```python
from build123d import *

# Parameters (mm, degrees)
SKETCH1_R           = 1.5
BOSS_EXTRUDE1_DEPTH = 3
SKETCH4_W           = 27
SKETCH4_H           = 30
BOSS_EXTRUDE2_DEPTH = 2
SKETCH5_W           = 26
SKETCH5_H           = 30
BOSS_EXTRUDE3_DEPTH = 14
FILLET1_R           = 3


with BuildPart() as part:
    # Sketch1 → Boss-Extrude1 (new body)
    with BuildSketch(Plane.XY):
        Polygon((-14.5, 16), (14.5, 16), (22, 0), (14.5, -16), (-14.5, -16), (-22, 0), align=None)
        with Locations((-18, 0)):
            Circle(SKETCH1_R, mode=Mode.SUBTRACT)
        with Locations((18, 0)):
            Circle(SKETCH1_R, mode=Mode.SUBTRACT)
    extrude(amount=BOSS_EXTRUDE1_DEPTH)

    # Sketch4 → Boss-Extrude2 (add)
    with BuildSketch(Plane.XY.offset(3)):
        Rectangle(SKETCH4_W, SKETCH4_H)
    extrude(amount=BOSS_EXTRUDE2_DEPTH)

    # Sketch5 → Boss-Extrude3 (add)
    with BuildSketch(Plane(origin=(0, 0, 0), x_dir=(-1, 0, 0), z_dir=(0, 0, -1))):
        Rectangle(SKETCH5_W, SKETCH5_H)
    extrude(amount=BOSS_EXTRUDE3_DEPTH)

    # Fillet1
    fillet1_edges = [part.edges().sort_by_distance(p)[0] for p in [
        (-14.5, 16, 1.5),
        (14.5, 16, 1.5),
        (22, 0, 1.5),
        (14.5, -16, 1.5),
        (-14.5, -16, 1.5),
        (-22, 0, 1.5),
        (13.5, -15, 4),
        (13.5, 15, 4),
        (-13.5, 15, 4),
        (-13.5, -15, 4),
        (-13, -15, -7),
        (-13, 15, -7),
        (13, 15, -7),
        (13, -15, -7),
    ]]
    fillet(fillet1_edges, radius=FILLET1_R)


solid = part.part
```
The listing builds one solid part. Answer for the finished solid, in the listing's coordinates (mm). A direction names the side the tool comes from. Round coordinates to 2 decimals unless told otherwise and drop trailing zeros. Order: outer loops, then holes, each group sorted by start corner. A loop starts at its lowest first (then second) coordinate and runs counter-clockwise, first axis right, second up. Notation, with made-up numbers: (-9.75, 64.5) -> (23.25, 64.5) arc R14 ccw to (23.25, 82.5) -> close; hole circle Ø6 at (29.25, 65). An arc over 180 degrees is marked (long way). Answer as CSV lines item,"result". Start each with the question number.
(1) Flat-ended cylindrical pins translate along their axes: pin 1 Ø1 at (x, y) = (15, 5) entering from +Z; pin 2 Ø5 at (y, z) = (12.5, -4) entering from -X; pin 3 Ø11 at (x, z) = (-4, -6.5) entering from +Y. Find the tip coordinate at first contact, or state that the pin passes through.
(2) Find the intervals of material crossed by probe 1 along Z at (x, y) = (15, 2.5); probe 2 along X at (y, z) = (3, 4.25); probe 3 along X at (y, z) = (5, -1), in increasing order. Write a range as from..to.
(3) The part is cut by section C-C (y = -8). Determine the outline of the cut face in (x, z).
(4) The part is cut by section D-D (z = -3). Determine the outline of the cut face in (x, y), then the cut area to 3 significant figures.
(5) For a pull along X with two mould halves and no side action, classify faces 1 (the face through (0, -15, -7)), 2 (the face through (16.5, 0.07, 1.48)), 3 (the face through (12.1, 14.14, -7.1)) as +X half, -X half, draft (parallel to the pull), parting line (faces both ways), or undercut.
(6) The part is cut by section A-A (y = 0). Determine the outline of the cut face in (x, z), then the cut area to 3 significant figures.
(7) The part is cut by section B-B (x = 18). Determine the outline of the cut face in (y, z), then the cut area to 3 significant figures.
(8) A tool of negligible diameter and unlimited length cuts with its end or side. For faces 4 (the face through (0, -15, 4)), 5 (the face through (-13, 0, -7)), 6 (the face through (-13.5, 0, 4)), from which of +Z, -Z, +X, -X, +Y, -Y can it reach the whole face along a straight path? Write none if from no direction.
Evaluation:
1,pin 1,"z = 3"
1,pin 2,"x = -13"
1,pin 3,"y = 15"
2,probe 1,"0..3"
2,probe 2,"-13.5..13.5"
2,probe 3,"-13..13"
3,outline,"(-18.25, 0) -> (-13, 0) -> (-13, -14) -> (13, -14) -> (13, 0) -> (18.25, 0) -> (18.25, 3) -> (13.5, 3) -> (13.5, 5) -> (-13.5, 5) -> (-13.5, 3) -> (-18.25, 3) -> close"
4,outline,"(-13, -12) arc R3 ccw to (-10, -15) -> (10, -15) arc R3 ccw to (13, -12) -> (13, 12) arc R3 ccw to (10, 15) -> (-10, 15) arc R3 ccw to (-13, 12) -> close"
4,area,"772 mm²"
5,face 1,"draft"
5,face 2,"undercut"
5,face 3,"+X half"
6,outline,"(-21.69, 0) -> (-19.5, 0) -> (-19.5, 3) -> (-21.69, 3) -> close; (-16.5, 0) -> (-13, 0) -> (-13, -14) -> (13, -14) -> (13, 0) -> (16.5, 0) -> (16.5, 3) -> (13.5, 3) -> (13.5, 5) -> (-13.5, 5) -> (-13.5, 3) -> (-16.5, 3) -> close; (19.5, 0) -> (21.69, 0) -> (21.69, 3) -> (19.5, 3) -> close"
6,area,"530 mm²"
7,outline,"(-8.53, 0) -> (-1.5, 0) -> (-1.5, 3) -> (-8.53, 3) -> close; (1.5, 0) -> (8.53, 0) -> (8.53, 3) -> (1.5, 3) -> close"
7,area,"42.2 mm²"
8,face 4,"+Z, +X, -X, -Y"
8,face 5,"-Z, -X, +Y, -Y"
8,face 6,"+Z, -X, +Y, -Y"
